from build123d import *

# Parameters (mm, degrees)
F1_DEPTH = 121.158
F2_R     = 25.4


with BuildPart() as f1:
    # F0 (on Front) → F1 (new body)
    with BuildSketch(Plane.XZ):
        with BuildLine():
            Line((24.5343538996, 51.4227636158), (-49.995383161, 51.4227636158))
            ThreePointArc((-49.995383161, 51.4227636158), (-60.3509792514, -4.7259186533), (-12.7305146307, -36.2251922997))
            Line((-12.7305146307, -36.2251922997), (-12.7305146307, 15.5206499621))
            Line((-12.7305146307, 15.5206499621), (39.0153276312, 15.5206499621))
            ThreePointArc((39.0153276312, 15.5206499621), (35.2587247896, 34.876917455), (24.5343538996, 51.4227636158))
        make_face()
    extrude(amount=F1_DEPTH)

    # F2
    f2_edges = [f1.edges().sort_by_distance(p)[0] for p in [
        (-12.730515, -121.158, 51.422764),
    ]]
    fillet(f2_edges, radius=F2_R)


solid = f1.part
Model file for the job. Use its own axes, mm. A direction names the side the tool comes from. Give positions to 0.01 mm unless a question says otherwise; leave off trailing zeros. Loops run counter-clockwise (first coordinate to the right, second up) from the corner with the lowest first, then second, coordinate; pieces in that order, holes last.
1) Saw through at A-A (x = 8). Write the cut outline in (y, z), plus the area to 3 significant figures.
2) Wall check: line 1 (Z direction, x = 6, y = -83); line 2 (Z direction, x = -14, y = -25.5); line 3 (Y direction, x = -33.5, z = 27). Give the ranges that are in metal, low to high.
3) Tool access for faces 1 (the flat face through (-12.731, -60, -11)), 2 (the cylindrical face through (-60.676, -59.731, -3.944)): list every direction of +Z, -Z, +X, -X, +Y, -Y with a clear straight run to the whole face (end or side of a thin tool).
4) Saw through at D-D (z = -7). Write the cut outline in (x, y), plus the area to 3 significant figures.
5) Flat gauge pins, fed straight in: pin 1 Ø10 at (y, z) = (-21.5, 33.5) entering from -X; pin 2 Ø1.5 at (y, z) = (-39, 29) entering from -X; pin 3 Ø15.5 at (x, y) = (22, -34) entering from -Z; pin 4 Ø8 at (x, z) = (23, 29.5) entering from -Y. Where does each tip first touch, or does it go through?
6) Saw through at C-C (z = -20). Write the cut outline in (x, y), plus the area to 3 significant figures.
7) Saw through at B-B (y = -85). Write the cut outline in (x, z).
Answer block:
1. outline: (-121.16, 15.52) - (0, 15.52) - (0, 51.42) - (-95.76, 51.42) arc R25.4 ccw to (-121.16, 26.02) - close
1. area: 4,210 mm2
2. line 1: z = 15.52 to 51.42
2. line 2: z = -36.21 to 51.42
2. line 3: y = -121.14 to 0
3. face 1: -Z, +X, +Y, -Y
3. face 2: -X, +Y, -Y
4. outline: (-59.32, -121.16) - (-12.73, -121.16) - (-12.73, 0) - (-59.32, 0) - close
4. area: 5,640 mm2
5. pin 1: stops at x = -62.82
5. pin 2: stops at x = -62.89
5. pin 3: stops at z = 15.52
5. pin 4: stops at y = -121.16
6. outline: (-50.36, -121.16) - (-12.73, -121.16) - (-12.73, 0) - (-50.36, 0) - close
6. area: 4,560 mm2
7. outline: (-50, 51.42) arc R51.75 ccw to (-12.73, -36.23) - (-12.73, 15.52) - (39.02, 15.52) arc R51.75 ccw to (24.53, 51.42) - close
